Source: three-view drawing plus pictorial views. Frame: mm from the lowest corner of the part. A direction names the side the tool comes from. Coordinates: 2 decimals unless noted, no trailing zeros. Order: outer loops, then holes, each group sorted by start corner. A loop starts at its lowest first (then second) coordinate and runs counter-clockwise, first axis right, second up. Notation, with made-up numbers: (-10.75, -2) -> (17.25, -2) arc R22 ccw to (17.25, 29) -> close; hole circle Ø10 at (8, 76.25). An arc over 180 degrees is marked (long way). Use one line per item in the form item = value. Start each with the question number.
1) Section query A-A on x = 3. Output: boundary loops of the cut face in (y, z), then the cut area to 3 significant figures.
2) Section query C-C on y = 0.75. Output: boundary loops of the cut face in (x, z).
3) Section query B-B on z = 3. Output: boundary loops of the cut face in (x, y).
4) Section query D-D on z = 4.4. Output: boundary loops of the cut face in (x, y), then the cut area to 3 significant figures.
5) Draft query along Z for the marked faces 3, 4 and 5. Return one class per face: pulls with the +Z half, pulls with the -Z half, needs draft (parallel to the pull), parting line crosses it, or undercut.
6) Access query for the marked faces 1 and 2. Directions: +Z, -Z, +X, -X, +Y, -Y. A direction counts if a zero-diameter tool reaches every point of the face in a straight line with its end or side. Return the directions, or none.
7) Ray query, line 1 along X through (y, z) = (1.3, 3); line 2 along Y through (x, z) = (3.05, 5.2); line 3 along Z through (x, y) = (2.6, 0.5). Return the intervals inside material, ascending.
8) Pin query (flat end, axial travel): pin 1 (0.6 mm diameter, centred on x = 3, z = 3, fed in from -Y); pin 2 (1.5 mm diameter, centred on y = 6, z = 1, fed in from -X); pin 3 (1.5 mm diameter, centred on x = 0.5, y = 2.5, fed in from +Z). Return the tip coordinate at first contact, or that it passes through.
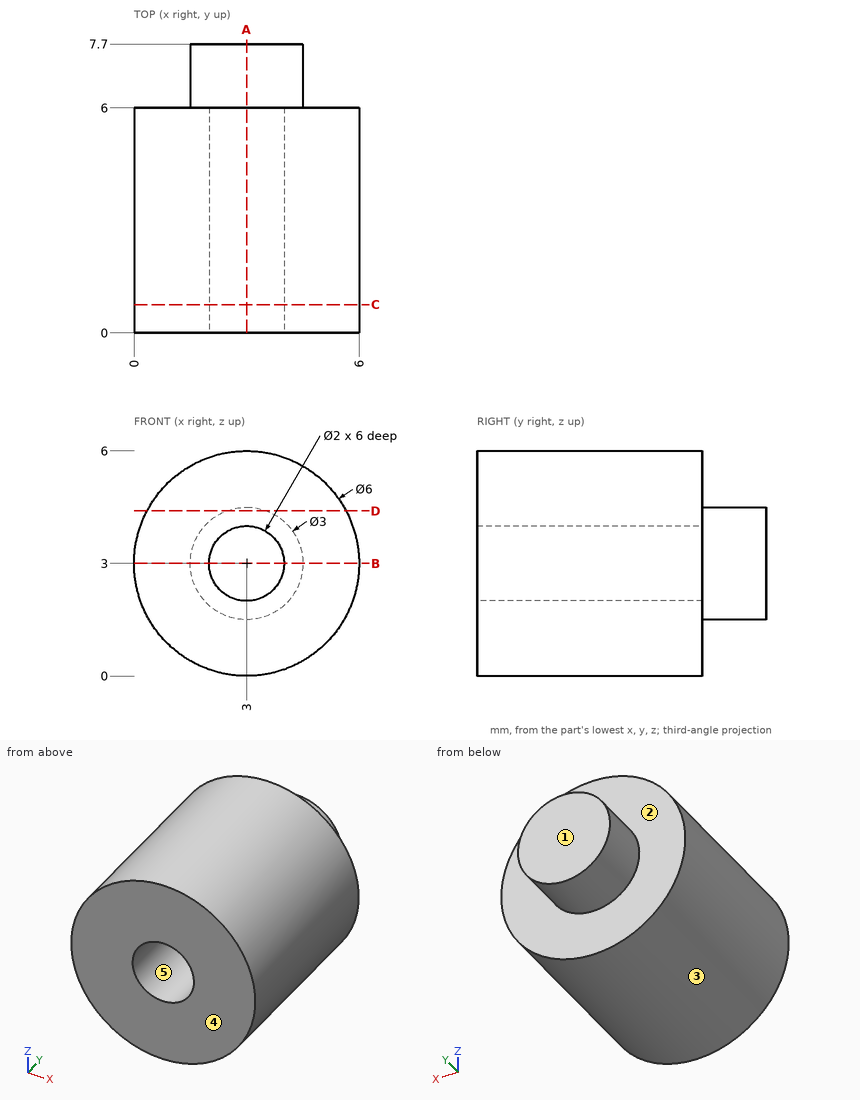
Answers below:
q1.outline = (0, 0) -> (6, 0) -> (6, 1.5) -> (7.7, 1.5) -> (7.7, 4.5) -> (6, 4.5) -> (6, 6) -> (0, 6) -> (0, 4) -> (6, 4) -> (6, 2) -> (0, 2) -> close
q1.area = 29.1 mm^2
q2.outline = circle Ø6 at (3, 3); hole circle Ø2 at (3, 3)
q3.outline = (0, 0) -> (2, 0) -> (2, 6) -> (4, 6) -> (4, 0) -> (6, 0) -> (6, 6) -> (4.5, 6) -> (4.5, 7.7) -> (1.5, 7.7) -> (1.5, 6) -> (0, 6) -> close
q4.outline = (0.35, 0) -> (5.65, 0) -> (5.65, 6) -> (3.54, 6) -> (3.54, 7.7) -> (2.46, 7.7) -> (2.46, 6) -> (0.35, 6) -> close
q4.area = 33.7 mm^2
q5.face_3 = parting line crosses it
q5.face_4 = needs draft
q5.face_5 = undercut
q6.face_1 = +Z, -Z, +X, -X, +Y
q6.face_2 = +Y
q7.line_1 = 0 to 2, 4 to 6
q7.line_2 = 0 to 6
q7.line_3 = 0.03 to 2.08, 3.92 to 5.97
q8.pin_1 = 6
q8.pin_2 = 0.27
q8.pin_3 = 5.44
